Geometry check sheet. Reference: the model listing, model coordinates, mm. A direction names the side the tool comes from. Give positions to 0.01 mm unless a question says otherwise; leave off trailing zeros. Loops run counter-clockwise (first coordinate to the right, second up) from the corner with the lowest first, then second, coordinate; pieces in that order, holes last.
1. Cross-section at D-D, the plane y = 3. Record the cut outline in (x, z).
2. Cross-section at A-A, the plane z = 1.95. Record the cut outline in (x, y).
3. Material ranges on L1, parallel to Y at x = 0, z = 5.05; L2, parallel to Y at x = -1, z = 1.2; L3, parallel to Z at x = -1.5, y = 1, recorded low to high.
4. Release check for a two-part mould opening along Y. For faces 3 (the flat face through (-2.774, -0.844, 1.479)), 4 (the cylindrical face through (4.72, 1.49, 2.91)), 5 (the flat face through (3.2, 0.1, 0)) record: +Y half, -Y half, draft (parallel to the pull), parting line (faces both ways), or undercut.
5. Cross-section at B-B, the plane x = 1.25. Record the cut outline in (y, z).
6. Go/stop test with flat-tipped pins: pin 1 Ø2.5 at (x, y) = (0, 0) entering from -Z; pin 2 Ø2 at (y, z) = (1.5, 5) entering from +X. Record where each tip stops, or that it passes through.
7. Tool access check on faces 1 (the flat face through (-0.656, -2.825, 1.479)), 2 (the cylindrical face through (1.27, -0.97, 4.43)). Record the directions out of +Z, -Z, +X, -X, +Y, -Y that give a thin tool (end or side, any length) a straight path to the whole face; none if there is none.
8. Cross-section at C-C, the plane y = 0. Record the cut outline in (x, z).
from build123d import *

# Parameters (mm, degrees)
ESQUISSE1_R             = 4.95
BOSS_EXTRU_1_DEPTH      = 5.9
ESQUISSE2_R             = 1.6
ENL_V_MAT_EXTRU_1_DEPTH = 5.9
ENL_V_MAT_EXTRU_2_DEPTH = 3


with BuildPart() as part:
    # Esquisse1 → Boss.-Extru.1 (new body)
    with BuildSketch(Plane.XY):
        Circle(ESQUISSE1_R)
    extrude(amount=BOSS_EXTRU_1_DEPTH)

    # Esquisse2 → Enlèv. mat.-Extru.1 (cut)
    with BuildSketch(Plane(origin=(0, 0, 0), x_dir=(-1, 0, 0), z_dir=(0, 0, -1))):
        Circle(ESQUISSE2_R)
    extrude(amount=-ENL_V_MAT_EXTRU_1_DEPTH, mode=Mode.SUBTRACT)

    # Esquisse3 → Enlèv. mat.-Extru.2 (cut)
    with BuildSketch(Plane(origin=(0, 0, 0), x_dir=(-1, 0, 0), z_dir=(0, 0, -1))):
        Polygon((-0.949092992, -3.211316837), (2.306535464, -2.42759706), (3.255628456, 0.783719777), (0.949092992, 3.211316837), (-2.306535464, 2.42759706), (-3.255628456, -0.783719777), align=None)
    extrude(amount=-ENL_V_MAT_EXTRU_2_DEPTH, mode=Mode.SUBTRACT)


solid = part.part
Result:
1. outline: (-3.94, 0) - (-1.15, 0) - (-1.15, 3) - (-0.07, 3) - (-0.07, 0) - (3.94, 0) - (3.94, 5.9) - (-3.94, 5.9) - close
2. outline: circle Ø9.9 at (0, 0); hole (-3.26, 0.78) - (-2.31, -2.43) - (0.95, -3.21) - (3.26, -0.78) - (2.31, 2.43) - (-0.95, 3.21) - close
3. L1: y = -4.95 to -1.6, 1.6 to 4.95
3. L2: y = -4.85 to -2.74, 3.16 to 4.85
3. L3: z = 3 to 5.9
4. face 3: undercut
4. face 4: parting line
4. face 5: draft
5. outline: (-4.79, 0) - (-2.89, 0) - (-2.89, 3) - (-1, 3) - (-1, 5.9) - (-4.79, 5.9) - close; (1, 3) - (2.68, 3) - (2.68, 0) - (4.79, 0) - (4.79, 5.9) - (1, 5.9) - close
6. pin 1: passes through
6. pin 2: stops at x = 4.92
7. face 1: -Z
7. face 2: +Z, -Z
8. outline: (-4.95, 0) - (-3.02, 0) - (-3.02, 3) - (-1.6, 3) - (-1.6, 5.9) - (-4.95, 5.9) - close; (1.6, 3) - (3.02, 3) - (3.02, 0) - (4.95, 0) - (4.95, 5.9) - (1.6, 5.9) - close
